from build123d import *

# Parameters (mm, degrees)
SKETCH1_W            = 99
SKETCH1_H            = 85
BOSS_EXTRUDE1_DEPTH  = 40
SKETCH2_W            = 88.5
SKETCH2_H            = 85
CUT_EXTRUDE1_DEPTH   = 31.5
SKETCH5_R            = 4.5
CUT_EXTRUDE3_DEPTH   = 3.3
SKETCH6_R            = 2.45
CUT_EXTRUDE4_DEPTH   = 5.2
SKETCH16_R           = 1.45
CUT_EXTRUDE6_DEPTH   = 93.75
SKETCH17_R           = 5
BOSS_EXTRUDE2_DEPTH  = 15
SKETCH18_W           = 10
SKETCH18_H           = 20
BOSS_EXTRUDE3_DEPTH  = 5
BOSS_EXTRUDE4_DEPTH  = 11
SKETCH20_W           = 15
SKETCH20_H           = 26.5
CUT_EXTRUDE7_DEPTH   = 93.75
FILLET1_R            = 10
FILLET2_R            = 5
FILLET1_OF_MIRROR3_R = 10
FILLET2_OF_MIRROR3_R = 5
SKETCH21_W           = 10
SKETCH21_H           = 20
BOSS_EXTRUDE5_DEPTH  = 5
BOSS_EXTRUDE7_DEPTH  = 11


with BuildPart() as part:
    # Sketch1 → Boss-Extrude1 (new body)
    with BuildSketch(Plane(origin=(0, 0, 0), x_dir=(1, 0, 0), z_dir=(0, 1, 0))):
        Rectangle(SKETCH1_W, SKETCH1_H)
    extrude(amount=BOSS_EXTRUDE1_DEPTH)

    # Sketch2 → Cut-Extrude1 (cut)
    with BuildSketch(Plane(origin=(0, 40, 0), x_dir=(1, 0, 0), z_dir=(0, 1, 0))):
        Rectangle(SKETCH2_W, SKETCH2_H)
    extrude(amount=-CUT_EXTRUDE1_DEPTH, mode=Mode.SUBTRACT)

    # Sketch5 → Cut-Extrude3 (cut)
    with BuildSketch(Plane(origin=(0, 8.5, 0), x_dir=(1, 0, 0), z_dir=(0, 1, 0))):
        with Locations((-39.5, 35)):
            Circle(SKETCH5_R)
        with Locations((9.5, 35)):
            Circle(SKETCH5_R)
        with Locations((-39.5, -35)):
            Circle(SKETCH5_R)
        with Locations((9.5, -35)):
            Circle(SKETCH5_R)
    extrude(amount=-CUT_EXTRUDE3_DEPTH, mode=Mode.SUBTRACT)

    # Sketch6 → Cut-Extrude4 (cut)
    with BuildSketch(Plane(origin=(0, 5.2, 0), x_dir=(1, 0, 0), z_dir=(0, 1, 0))):
        with Locations((-39.5, 35)):
            Circle(SKETCH6_R)
        with Locations((9.5, 35)):
            Circle(SKETCH6_R)
        with Locations((9.5, -35)):
            Circle(SKETCH6_R)
        with Locations((-39.5, -35)):
            Circle(SKETCH6_R)
    extrude(amount=-CUT_EXTRUDE4_DEPTH, mode=Mode.SUBTRACT)

    # Sketch16 → Cut-Extrude6 (cut)
    with BuildSketch(Plane.ZY.offset(49.5)):
        with Locations((-29, 31.4)):
            Circle(SKETCH16_R)
        with Locations((16.5, 31.4)):
            Circle(SKETCH16_R)
    cut_extrude6 = extrude(amount=-CUT_EXTRUDE6_DEPTH, mode=Mode.SUBTRACT)

    # Mirror1: Cut-Extrude6 across plane
    add(cut_extrude6.mirror(Plane(origin=(0, 0, 0), x_dir=(0, 0, 1), z_dir=(1, 0, 0))), mode=Mode.SUBTRACT)

    # Sketch17 → Boss-Extrude2 (add)
    with BuildSketch(Plane(origin=(49.5, 0, 0), x_dir=(0, 0, -1), z_dir=(1, 0, 0))):
        with Locations((-8.6, 20)):
            Circle(SKETCH17_R)
        with Locations((21.1, 20)):
            Circle(SKETCH17_R)
    extrude(amount=BOSS_EXTRUDE2_DEPTH)

    # Sketch18 → Boss-Extrude3 (add)
    with BuildSketch(Plane(origin=(64.5, 0, 0), x_dir=(0, 0, -1), z_dir=(1, 0, 0))):
        with Locations((-8.6, 30)):
            Rectangle(SKETCH18_W, SKETCH18_H)
    extrude(amount=-BOSS_EXTRUDE3_DEPTH)

    # Sketch19 → Boss-Extrude4 (add)
    with BuildSketch(Plane(origin=(64.5, 0, 0), x_dir=(0, 0, -1), z_dir=(1, 0, 0))):
        with BuildLine():
            Line((-13.6, 40), (-3.6, 40))
            ThreePointArc((-3.6, 40), (-8.6, 35), (-13.6, 40))
        make_face()
    extrude(amount=-BOSS_EXTRUDE4_DEPTH)

    # Sketch20 → Cut-Extrude7 (cut)
    with BuildSketch(Plane.ZY.offset(49.5)):
        with Locations((35, 26.75)):
            Rectangle(SKETCH20_W, SKETCH20_H)
    cut_extrude7 = extrude(amount=-CUT_EXTRUDE7_DEPTH, mode=Mode.SUBTRACT)

    # Fillet1
    fillet1_edges = [part.edges().sort_by_distance(p)[0] for p in [
        (-46.875, 40, 27.5),
    ]]
    fillet(fillet1_edges, radius=FILLET1_R)

    # Fillet2
    fillet2_edges = [part.edges().sort_by_distance(p)[0] for p in [
        (-46.875, 13.5, 42.5),
    ]]
    fillet(fillet2_edges, radius=FILLET2_R)

    # Mirror3: Cut-Extrude7 across plane
    add(cut_extrude7.mirror(Plane(origin=(0, 0, 0), x_dir=(0, 0, 1), z_dir=(1, 0, 0))), mode=Mode.SUBTRACT)

    # Fillet1 of Mirror3
    fillet1_of_mirror3_edges = [part.edges().sort_by_distance(p)[0] for p in [
        (46.875, 40, 27.5),
    ]]
    fillet(fillet1_of_mirror3_edges, radius=FILLET1_OF_MIRROR3_R)

    # Fillet2 of Mirror3
    fillet2_of_mirror3_edges = [part.edges().sort_by_distance(p)[0] for p in [
        (46.875, 13.5, 42.5),
    ]]
    fillet(fillet2_of_mirror3_edges, radius=FILLET2_OF_MIRROR3_R)

    # Sketch21 → Boss-Extrude5 (add)
    with BuildSketch(Plane(origin=(64.5, 0, 0), x_dir=(0, 0, -1), z_dir=(1, 0, 0))):
        with Locations((21.1, 30)):
            Rectangle(SKETCH21_W, SKETCH21_H)
    extrude(amount=-BOSS_EXTRUDE5_DEPTH)

    # Sketch23 → Boss-Extrude7 (add)
    with BuildSketch(Plane(origin=(64.5, 0, 0), x_dir=(0, 0, -1), z_dir=(1, 0, 0))):
        with BuildLine():
            Line((16.1, 40), (26.1, 40))
            ThreePointArc((26.1, 40), (21.1, 35), (16.1, 40))
        make_face()
    extrude(amount=-BOSS_EXTRUDE7_DEPTH)


solid = part.part
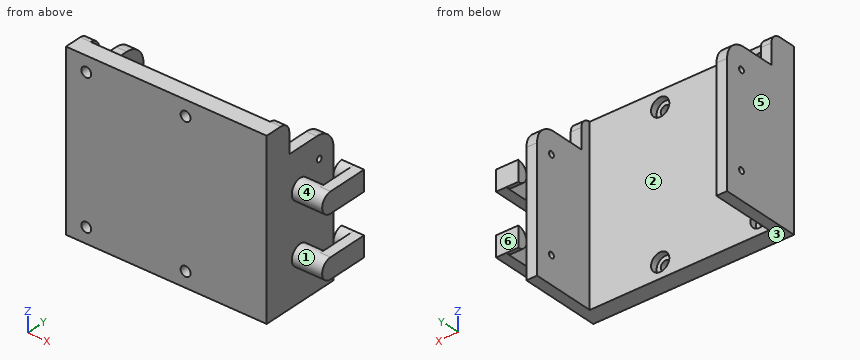
Could you check a few things on this model? Use its own coordinates, in mm. Face numbers are marked on the shaded views. A direction names the side the tool comes from. Coordinates: 2 decimals unless noted, no trailing zeros. Write each loop counter-clockwise with the first axis right and the second up, starting at its lowest first coordinate (ties: lowest second). Pieces come first, ordered by that corner, then holes. Notation, with made-up numbers: (78.5, -19) - (100.5, -19) arc R21 cw to (100.5, -9) - close; hole circle Ø7 at (82.25, 44). An arc over 180 degrees is marked (long way). Put each result on its own line as item: value. Start each with the question number.
Q1. I want a section at C-C on x = 2.5. Write out the boundary of the cut face in (y, z).
Q2. Which directions (+Z, -Z, +X, -X, +Y, -Y) give clear straight access to the entire face, cutting with the end or side of a thin tool? Please do the marked faces 1, 2 and 3.
Q3. I want a section at A-A on z = -35. Write out the boundary of the cut face in (x, y).
Q4. Please list where these lines run through material, in increasing order: L1, parallel to Z at x = -39.5, y = 3.1; L2, parallel to X at y = 2.2, z = -35; L3, parallel to X at y = 6.1, z = 35.
Q5. I'm going to push flat-ended pins straight in: P1, Ø6.5, axis at x = -39.5, z = 35, coming from the -Y side; P2, Ø4, axis at y = 31.4, z = 16.5, coming from the +X side; P3, Ø6, axis at x = -48, y = 21.5, coming from the +Z side; P4, Ø2.5, axis at x = -45.5, z = 31, coming from the +Y side. Where does each tip first touch, or does it pass through?
Q6. Thinking about a two-plate mould opening in X: for the marked faces 4, 5 and 6, which applies, pulls with the +X half, pulls with the -X half, needs draft (parallel to the pull), parting line crosses it, or undercut?
Q7. I want a section at B-B on z = -13. Write out the boundary of the cut face in (x, y).
Q8. I want a section at D-D on z = 8.6. Write out the boundary of the cut face in (x, y).
Checks:
1. outline: (0, -42.5) - (8.5, -42.5) - (8.5, 42.5) - (0, 42.5) - close
2. face 1: none
2. face 2: +Z, -Z, +Y
2. face 3: -Z, +X, -X, +Y, -Y
3. outline: (-49.5, 0) - (-41.95, 0) - (-41.95, 5.2) - (-44, 5.2) - (-44, 8.5) - (-44.25, 8.5) - (-44.25, 40) - (-49.5, 40) - close; (-37.05, 0) - (7.05, 0) - (7.05, 5.2) - (5, 5.2) - (5, 8.5) - (-35, 8.5) - (-35, 5.2) - (-37.05, 5.2) - close; (11.95, 0) - (49.5, 0) - (49.5, 40) - (44.25, 40) - (44.25, 8.5) - (14, 8.5) - (14, 5.2) - (11.95, 5.2) - close
4. L1: -42.5 to -37.45, -32.55 to 32.55, 37.45 to 42.5
4. L2: -49.5 to -41.95, -37.05 to 7.05, 11.95 to 49.5
4. L3: -49.5 to -44, -35 to 5, 14 to 49.5
5. P1: y = 0
5. P2: x = 49.5
5. P3: z = 27.5
5. P4: y = 13.5
6. face 4: undercut
6. face 5: pulls with the -X half
6. face 6: needs draft
7. outline: (-49.5, 0) - (49.5, 0) - (49.5, 40) - (44.25, 40) - (44.25, 8.5) - (-44.25, 8.5) - (-44.25, 40) - (-49.5, 40) - close
8. outline: (-49.5, 0) - (49.5, 0) - (49.5, 15) - (64.5, 15) - (64.5, 40) - (53.5, 40) - (53.5, 35) - (59.5, 35) - (59.5, 25) - (49.5, 25) - (49.5, 40) - (44.25, 40) - (44.25, 8.5) - (-44.25, 8.5) - (-44.25, 40) - (-49.5, 40) - close
